Autodesk Inventor part; units mm, degrees
ref_plane "作業平面2" through (0, 0, 0) normal (1, 0, 0) x (0, 0, -1)
ref_plane "YZ Plane" through (0, 0, 0) normal (1, 0, 0) x (0, 1, 0)
ref_plane "XZ Plane" through (0, 0, 0) normal (0, 1, 0) x (-1, 0, 0)
sketch "スケッチ1" plane through (0, 0, 0) normal (0, 1, 0) x (-1, 0, 0)
  arc A0 (0.9, 0) -> (-0.9, 0) centre (0, 0) ccw
  arc A1 (-0.9, -4) -> (0.9, -4) centre (0, -4) ccw
  line L0 (0, 0) -> (0, -4) construction
  line L1 (-0.9, -4) -> (-0.9, 0)
  line L2 (0.9, -4) -> (0.9, 0)
  arc A2 (-2.5, -4) -> (2.5, -4) centre (0, -4) ccw
  line L3 (-2.5, -4) -> (-2.5, 0)
  arc A3 (2.5, 0) -> (-2.5, 0) centre (0, 0) ccw
  line L4 (2.5, 0) -> (2.5, -4)
  line L5 (-2.5, -2.5) -> (-7.75, -2.5)
  line L6 (-7.75, -2.5) -> (-7.75, 2.5)
  line L7 (-7.75, 2.5) -> (-2.75, 2.5)
  line L8 (-2.75, -2.5) -> (-7.75, -2.5)
  line L9 (-7.75, -2.5) -> (-7.75, 2.5)
  line L10 (-7.75, 2.5) -> (-2.75, 2.5)
  line L11 (-2.75, 2.5) -> (-2.75, -2.5)
  line L12 (-2.75, 2.5) -> (0, 2.5)
  point P0 (-5.25, -2.5)
  point P1 (-3.4, 2.5)
  point P2 (0, 2.5)
  dimension "d0" = 1.8
  dimension "d1" = 4
  dimension "d2" = 1.6
  dimension "d40" = 5
  dimension "d41" = 5.25
  dimension "d42" = 5
extrude "押し出し1" add sketch "スケッチ1" along normal blind 2
extrude "押し出し4" add sketch "スケッチ1" against normal blind 7.3 contours L5 L6 L7 L11
sketch "スケッチ6" plane through (7.75, 2, 2.5) normal (1, 0, 0) x (0, 0, -1)
  line L0 (5, -9.3) -> (0, -9.3)
  point P0 (2.5, -2)
  point P1 (2.5, -7.1)
  point P2 (2.5, -9.3)
  dimension "d43" = 2.2
hole "穴3" at (7.75, -5.1, 0) direction (-1, 0, 0) diameter 2.2 end through all
fillet "フィレット3" radius 1 1 edges at (2.75, 0, 0)
ref_plane "作業平面2" through (0, 0, 0) normal (1, 0, 0) x (0, 0, -1)
chamfer "面取り1" distance 1 angle 45 2 edges at (2.75, -7.3, 0) (7.75, -7.3, 0)
sketch "スケッチ7" plane through (0, -7.3, 0) normal (0, -1, 0) x (1, 0, 0)
  line L0 (6.75, 2.5) -> (6.75, -2.5)
  line L1 (3.75, -2.5) -> (3.75, 2.5)
  line L2 (6.75, 0.75) -> (3.75, 0.75)
  line L3 (3.75, 0.75) -> (3.75, -0.75)
  line L4 (3.75, -0.75) -> (6.75, -0.75)
  line L5 (6.75, -0.75) -> (6.75, 0.75)
  point P0 (0, 0)
  point P1 (6.75, 0)
  point P2 (6.75, 0.75)
  point P3 (3.75, 0.75)
  dimension "d55" = 1.5
extrude "押し出し5" add sketch "スケッチ7" along normal blind 1
properties part number "om_Drop_10g_L" material "ABS プラスチック"
The listing builds one solid part. Answer for the finished solid, in the listing's coordinates (mm). A direction names the side the tool comes from. Give positions to 0.01 mm unless a question says otherwise; leave off trailing zeros. Loops run counter-clockwise (first coordinate to the right, second up) from the corner with the lowest first, then second, coordinate; pieces in that order, holes last. Notation, with made-up numbers: (65.25, 55.25) - (113.25, 55.25) arc R8 cw to (113.25, 66.25) - close; hole circle Ø5 at (83, 47.25). An arc over 180 degrees is marked (long way). Return JSON: item names as keys, results as strings. Group by question number.
1. Determine the mould class of faces 5 (the cylindrical face through (0, 1, 0.9)), 6 (the flat face through (5, -3, 2.5)), 7 (the flat face through (7.75, -2, 0)) for opening direction X: pulls with the +X half, pulls with the -X half, needs draft (parallel to the pull), parting line crosses it, or undercut.
2. Given pin 1 Ø4 at (y, z) = (-7, -3.5) entering from -X; pin 2 Ø2 at (x, y) = (3, -3.5) entering from -Z; pin 3 Ø1.9 at (x, z) = (5, 2) entering from -Y, each flat-ended and moving along its own axis, determine where each tip first touches the part or whether it passes through.
3. Find section C-C (x = 6.25). Write down the section's boundary in (y, z).
4. Find section A-A (x = -0.25). Write down the section's boundary in (y, z), then the cut area to 3 significant figures.
5. Which of the six approach directions +Z, -Z, +X, -X, +Y, -Y give full straight-line access (tool end or side, diameter ignored) to faces 1 (the flat face through (5, -8, 0.75)), 2 (the flat face through (3.75, -8, 0)), 3 (the flat face through (5, -7.3, -2)), 4 (the flat face through (2.5, 1, -3))?
6. Find section D-D (z = 1.25). Write down the section's boundary in (x, y).
7. Straight lines are drawn through the part: line 1 (Y direction, x = 5.85, z = 0); line 2 (Z direction, x = 5.3, y = -5.1); line 3 (X direction, y = 1.5, z = -0.75). For each, find the intervals that lie inside material, in ascending order. Write a range as [from, to].
8. Find section B-B (y = -5.1). Write down the section's boundary in (x, z).
Verdict:
{
 "1": {"face 5": "undercut", "face 6": "needs draft", "face 7": "pulls with the +X half"},
 "2": {"pin 1": "stops at x = 2.75", "pin 2": "stops at z = -2.5", "pin 3": "stops at y = -7.3"},
 "3": {"outline": "(-8.3, -0.75) - (-7.3, -0.75) - (-7.3, -2.5) - (2, -2.5) - (2, 2.5) - (-7.3, 2.5) - (-7.3, 0.75) - (-8.3, 0.75) - close; hole circle Ø2.2 at (-5.1, 0)"},
 "4": {"outline": "(0, -6.49) - (2, -6.49) - (2, -4.86) - (0, -4.86) - close; (0, 0.86) - (2, 0.86) - (2, 2.49) - (0, 2.49) - close", "area": "6.49 mm^2"},
 "5": {"face 1": "+Z, +X, -X, -Y", "face 2": "+Z, -Z, -X, -Y", "face 3": "-Z, +X, -X, -Y", "face 4": "-Z, +X, +Y, -Y"},
 "6": {"outline": "(-2.17, 0) - (1.75, 0) arc R1 cw to (2.75, -1) - (2.75, -6.3) - (3.75, -7.3) - (6.75, -7.3) - (7.75, -6.3) - (7.75, 2) - (-2.17, 2) - close"},
 "7": {"line 1": "y = [-8.3, -6.2], [-4, 2]", "line 2": "z = [-2.5, -1.1], [1.1, 2.5]", "line 3": "x = [-2.5, -0.9], [0.9, 7.75]"},
 "8": {"outline": "(2.75, -2.5) - (7.75, -2.5) - (7.75, -1.1) - (2.75, -1.1) - close; (2.75, 1.1) - (7.75, 1.1) - (7.75, 2.5) - (2.75, 2.5) - close"}
}
